Check sheet for the modelled part. Datum: model origin and axes. Units: mm. Coordinates: 2 decimals unless noted, no trailing zeros. Write each loop counter-clockwise with the first axis right and the second up, starting at its lowest first coordinate (ties: lowest second). Pieces come first, ordered by that corner, then holes. Notation, with made-up numbers: (9.5, 49.25) -> (38.5, 49.25) arc R24 ccw to (38.5, 59.25) -> close; hole circle Ø3 at (35.25, 70). An arc over 180 degrees is marked (long way). Put each result on its own line as item: value.
```python
from build123d import *

# Parameters (mm, degrees)
SKETCH1_R                    = 101.219
SKETCH1_R_2                  = 73.8124
BOSS_EXTRUDE1_DEPTH          = 22.352
SKETCH2_R                    = 76.454
CUT_EXTRUDE1_DEPTH           = 9.652
CHAMFER1_SIZE                = 0.762
SKETCH3_R                    = 4.2164
CUT_EXTRUDE2_DEPTH           = 23.352
CHAMFER2_SIZE                = 0.381
CIRPATTERN1_COUNT            = 20
CHAMFER2_OF_CIRPATTERN1_SIZE = 0.381
CUT_EXTRUDE3_DEPTH           = 0.79375


with BuildPart() as part:
    # Sketch1 → Boss-Extrude1 (new body)
    with BuildSketch(Plane(origin=(0, 0, 0), x_dir=(1, 0, 0), z_dir=(0, 1, 0))):
        Circle(SKETCH1_R)
        Circle(SKETCH1_R_2, mode=Mode.SUBTRACT)
    extrude(amount=BOSS_EXTRUDE1_DEPTH)

    # Sketch2 → Cut-Extrude1 (cut)
    with BuildSketch(Plane(origin=(0, 22.352, 0), x_dir=(-1, 0, 0), z_dir=(0, -1, 0))):
        Circle(SKETCH2_R)
    extrude(amount=CUT_EXTRUDE1_DEPTH, mode=Mode.SUBTRACT)

    # Chamfer1
    chamfer1_edges = [part.edges().sort_by_distance(p)[0] for p in [
        (76.454, 22.352, 0),
        (-101.219, 0, 0),
        (-101.219, 22.352, 0),
    ]]
    chamfer(chamfer1_edges, length=CHAMFER1_SIZE)

    # Sketch4 → Cut-Revolve1 (revolve, cut)
    with BuildSketch(Plane.XY):
        Polygon((-85.725, 0), (-85.725, 1.6256), (-83.058, 0.6604), (-83.058, 1.27), (0, 1.27), (0, 0), align=None)
    revolve(axis=Axis((0, 22.352, 0), (0, -1, 0)), mode=Mode.SUBTRACT)

    # Sketch3 → Cut-Extrude2 (cut, through all)
    with BuildSketch(Plane(origin=(0, 22.352, 0), x_dir=(1, 0, 0), z_dir=(0, 1, 0))):
        with Locations((-14.161323808, 89.411079645)):
            Circle(SKETCH3_R)
    cut_extrude2 = extrude(amount=-CUT_EXTRUDE2_DEPTH, mode=Mode.SUBTRACT)

    # Chamfer2
    chamfer2_edges = [part.edges().sort_by_distance(p)[0] for p in [
        (-18.377723808, 0, -89.411079645),
        (-18.377723808, 22.352, -89.411079645),
    ]]
    chamfer(chamfer2_edges, length=CHAMFER2_SIZE)

    # CirPattern1: Cut-Extrude2 ×20 about axis
    cirpattern1_axis = Axis((0, 0, 0), (0, 1, 0))
    for i in range(1, CIRPATTERN1_COUNT):
        add(cut_extrude2.rotate(cirpattern1_axis, i * 360 / CIRPATTERN1_COUNT), mode=Mode.SUBTRACT)

    # Chamfer2 of CirPattern1
    chamfer2_of_cirpattern1_edges = [part.edges().sort_by_distance(p)[0] for p in [
        (-45.107797079, 0, -79.355960951),
        (-45.107797079, 22.352, -79.355960951),
        (-67.422404886, 0, -61.532927893),
        (-67.422404886, 22.352, -61.532927893),
        (-83.137237944, 0, -37.686623128),
        (-83.137237944, 22.352, -37.686623128),
        (-90.7140189, 0, -10.151289113),
        (-90.7140189, 22.352, -10.151289113),
        (-89.411079645, 0, 18.377723808),
        (-89.411079645, 22.352, 18.377723808),
        (-79.355960951, 0, 45.107797079),
        (-79.355960951, 22.352, 45.107797079),
        (-61.532927893, 0, 67.422404886),
        (-61.532927893, 22.352, 67.422404886),
        (-37.686623128, 0, 83.137237944),
        (-37.686623128, 22.352, 83.137237944),
        (-10.151289113, 0, 90.7140189),
        (-10.151289113, 22.352, 90.7140189),
        (18.377723808, 0, 89.411079645),
        (18.377723808, 22.352, 89.411079645),
        (45.107797079, 0, 79.355960951),
        (45.107797079, 22.352, 79.355960951),
        (67.422404886, 0, 61.532927893),
        (67.422404886, 22.352, 61.532927893),
        (83.137237944, 0, 37.686623128),
        (83.137237944, 22.352, 37.686623128),
        (90.7140189, 0, 10.151289113),
        (90.7140189, 22.352, 10.151289113),
        (89.411079645, 0, -18.377723808),
        (89.411079645, 22.352, -18.377723808),
        (79.355960951, 0, -45.107797079),
        (79.355960951, 22.352, -45.107797079),
        (61.532927893, 0, -67.422404886),
        (61.532927893, 22.352, -67.422404886),
        (37.686623128, 0, -83.137237944),
        (37.686623128, 22.352, -83.137237944),
        (10.151289113, 0, -90.7140189),
        (10.151289113, 22.352, -90.7140189),
    ]]
    chamfer(chamfer2_of_cirpattern1_edges, length=CHAMFER2_OF_CIRPATTERN1_SIZE)

    # Sketch5 → Cut-Extrude3 (cut, symmetric)
    with BuildSketch(Plane.XY):
        Polygon((-85.354321688, 0.946996712), (-101.219, 1.778429271), (-101.219, -3.52623374), (-85.354321688, -3.52623374), align=None)
        Polygon((85.354321688, 0.946996712), (85.354321688, -3.52623374), (101.219, -3.52623374), (101.219, 1.778429271), align=None)
    extrude(amount=CUT_EXTRUDE3_DEPTH, both=True, mode=Mode.SUBTRACT)


solid = part.part
```
Q1. Cross-section at B-B (y = 5.5). State how many separate pieces and enclosed holes the cut face has, plus the area to 3 significant figures.
Recorded:
separate pieces: 1
enclosed holes: 21
area: 14,000 mm2
Q2. Depth check by flat-ended pin: P1, Ø0.5, axis at x = 91, y = 1, coming from the +Z side; P2, Ø6, axis at x = 17.5, y = 8.5, coming from the +Z side (3 decimals); P3, Ø9.5, axis at x = 64.01, z = 64.01, coming from the -Y side; P4, Ø4, axis at x = 5.5, y = 13.5, coming from the +Z side. Enter the tip coordinate at first touch or a pass-through.
Recorded:
P1: stops at z = 44.83
P2: stops at z = 100.175
P3: stops at y = 0
P4: stops at z = 101.16
Q3. Cross-section at A-A (x = 0). Record the cut outline in (y, z) (3 decimals).
Recorded:
outline: (0, -100.457) -> (0.762, -101.219) -> (21.59, -101.219) -> (22.352, -100.457) -> (22.352, -77.216) -> (21.59, -76.454) -> (12.7, -76.454) -> (12.7, -73.812) -> (1.27, -73.812) -> (1.27, -83.058) -> (0.66, -83.058) -> (1.626, -85.725) -> (0, -85.725) -> close; (0, 85.725) -> (1.626, 85.725) -> (0.66, 83.058) -> (1.27, 83.058) -> (1.27, 73.812) -> (12.7, 73.812) -> (12.7, 76.454) -> (21.59, 76.454) -> (22.352, 77.216) -> (22.352, 100.457) -> (21.59, 101.219) -> (0.762, 101.219) -> (0, 100.457) -> close
Q4. Material ranges on line 1 along X through (y, z) = (19.75, 0); line 2 along X through (y, z) = (7.5, 65); line 3 along Z through (x, y) = (65.5, 9), recorded low to high.
Recorded:
line 1: x = -101.22 to -76.45, 76.45 to 101.22
line 2: x = -77.59 to -68.11, -59.91 to -34.98, 34.98 to 59.91, 68.11 to 77.59
line 3: z = -77.17 to -67.96, -60.07 to -34.03, 34.03 to 60.07, 67.96 to 77.17
